from build123d import *

# Parameters (mm, degrees)
SKETCH1_W           = 160
SKETCH1_H           = 100
BOSS_EXTRUDE1_DEPTH = 50
SKETCH2_W           = 20
SKETCH2_H           = 40
CUT_EXTRUDE1_DEPTH  = 20
SKETCH3_W           = 30
SKETCH3_H           = 20
CUT_EXTRUDE2_DEPTH  = 20
SKETCH4_W           = 120
SKETCH4_H           = 60
CUT_EXTRUDE3_DEPTH  = 30
BOSS_EXTRUDE2_DEPTH = 30
SKETCH8_W           = 30
SKETCH8_H           = 40
BOSS_EXTRUDE3_DEPTH = 20


with BuildPart() as part:
    # Sketch1 → Boss-Extrude1 (new body)
    with BuildSketch(Plane.XY):
        with Locations((80, 50)):
            Rectangle(SKETCH1_W, SKETCH1_H)
    extrude(amount=BOSS_EXTRUDE1_DEPTH)

    # Sketch2 → Cut-Extrude1 (cut)
    with BuildSketch(Plane.XY.offset(50)):
        with Locations((10, 50)):
            Rectangle(SKETCH2_W, SKETCH2_H)
        with Locations((150, 50)):
            Rectangle(SKETCH2_W, SKETCH2_H)
    extrude(amount=-CUT_EXTRUDE1_DEPTH, mode=Mode.SUBTRACT)

    # Sketch3 → Cut-Extrude2 (cut)
    with BuildSketch(Plane(origin=(0, 0, 0), x_dir=(-1, 0, 0), z_dir=(0, 0, -1))):
        with Locations((-55, 50)):
            Rectangle(SKETCH3_W, SKETCH3_H)
        with Locations((-105, 50)):
            Rectangle(SKETCH3_W, SKETCH3_H)
    extrude(amount=-CUT_EXTRUDE2_DEPTH, mode=Mode.SUBTRACT)

    # Sketch4 → Cut-Extrude3 (cut)
    with BuildSketch(Plane.XY.offset(50)):
        with Locations((80, 50)):
            Rectangle(SKETCH4_W, SKETCH4_H)
    extrude(amount=-CUT_EXTRUDE3_DEPTH, mode=Mode.SUBTRACT)

    # Sketch5 → Boss-Extrude2 (add)
    with BuildSketch(Plane.XY.offset(50)):
        Polygon((80, 100), (80, 80), (140, 80), (140, 70), (160, 70), (160, 100), align=None)
        Polygon((80, 0), (80, 20), (140, 20), (140, 30), (160, 30), (160, 0), align=None)
    extrude(amount=BOSS_EXTRUDE2_DEPTH)

    # Sketch8 → Boss-Extrude3 (add)
    with BuildSketch(Plane.ZY.offset(-140)):
        with Locations((45, 50)):
            Rectangle(SKETCH8_W, SKETCH8_H)
    extrude(amount=-BOSS_EXTRUDE3_DEPTH)


solid = part.part
Check sheet for the modelled part. Datum: model origin and axes. Units: mm. A direction names the side the tool comes from. Round coordinates to 2 decimals unless told otherwise and drop trailing zeros. Loops run counter-clockwise (first coordinate to the right, second up) from the corner with the lowest first, then second, coordinate; pieces in that order, holes last. Notation, with made-up numbers: (60, 3.5) -> (114, 3.5) arc R33 cw to (114, 38.5) -> close; hole circle Ø10 at (69.5, 21). An arc over 180 degrees is marked (long way). Put each result on its own line as item: value. Start each with the question number.
1. Draft check along X on faces 1 (the face through (105, 40, 10)), 2 (the face through (55, 60, 10)), 3 (the face through (160, 51, 39)), 4 (the face through (119, 89, 80)). Enter one of: +X half, -X half, draft (parallel to the pull), parting line (faces both ways), or undercut.
2. Scan lines: probe 1 along X at (y, z) = (52.5, 19); probe 2 along Y at (x, z) = (92, 39); probe 3 along X at (y, z) = (41, 23). Record each from-to range of solid material in increasing order.
3. Gauge pin test, flat ends, axial feed: pin 1 (6 mm diameter, centred on x = 14.5, y = 55.5, fed in from +Z); pin 2 (8 mm diameter, centred on x = 24, y = 23, fed in from -Z); pin 3 (16 mm diameter, centred on y = 10.5, z = 69.5, fed in from -X); pin 4 (12 mm diameter, centred on x = 131, y = 38, fed in from +Z). Record the tip position at first contact, or that the pin passes through.
4. Section check A-A (x = 49.5). Enter the section's corners in (y, z), plus the area to 3 significant figures.
5. Section check C-C (y = 56). Enter the section's corners in (x, z), plus the area to 3 significant figures.
6. Access from +Z, -Z, +X, -X, +Y, -Y to the whole of each face (thin tool, end or side, straight path). Record for faces 5 (the face through (55, 40, 10)), 6 (the face through (150, 70, 70)), 7 (the face through (10, 50, 30)), 8 (the face through (80, 90, 65)), 9 (the face through (79, 50, 20)).
7. Section check D-D (x = 12). Enter the section's corners in (y, z).
8. Section check B-B (z = 22). Enter the section's corners in (x, y), plus the area to 3 significant figures.
Findings:
1. face 1: undercut
1. face 2: undercut
1. face 3: +X half
1. face 4: draft
2. probe 1: x = 0 to 40, 70 to 90, 120 to 160
2. probe 2: y = 0 to 20, 80 to 100
2. probe 3: x = 0 to 20, 140 to 160
3. pin 1: stops at z = 30
3. pin 2: stops at z = 0
3. pin 3: stops at x = 80
3. pin 4: stops at z = 20
4. outline: (0, 0) -> (40, 0) -> (40, 20) -> (20, 20) -> (20, 50) -> (0, 50) -> close; (60, 0) -> (100, 0) -> (100, 50) -> (80, 50) -> (80, 20) -> (60, 20) -> close
4. area: 2,800 mm^2
5. outline: (0, 0) -> (40, 0) -> (40, 20) -> (20, 20) -> (20, 30) -> (0, 30) -> close; (70, 0) -> (90, 0) -> (90, 20) -> (70, 20) -> close; (120, 0) -> (160, 0) -> (160, 60) -> (140, 60) -> (140, 20) -> (120, 20) -> close
5. area: 3,000 mm^2
6. face 5: +Z, -Z
6. face 6: +Z, +X, -X
6. face 7: +Z, -X
6. face 8: +Z, -X, +Y, -Y
6. face 9: +Z
7. outline: (0, 0) -> (100, 0) -> (100, 50) -> (70, 50) -> (70, 30) -> (30, 30) -> (30, 50) -> (0, 50) -> close
8. outline: (0, 0) -> (160, 0) -> (160, 100) -> (0, 100) -> close; hole (20, 20) -> (140, 20) -> (140, 80) -> (20, 80) -> close
8. area: 8,800 mm^2
